Model file for the job. Use its own axes, mm. A direction names the side the tool comes from. Give positions to 0.01 mm unless a question says otherwise; leave off trailing zeros. Loops run counter-clockwise (first coordinate to the right, second up) from the corner with the lowest first, then second, coordinate; pieces in that order, holes last. Notation, with made-up numbers: M -8,45 L 15,45 A15 ccw 15,56 Z; hole C -25.75,-32.5 d11. An arc over 180 degrees is marked long. Answer in a Markdown table with one row per item.
```python
from build123d import *

# Parameters (mm, degrees)
BOSS_EXTRUDE1_DEPTH = 22.5
SKETCH2_W           = 6.85
SKETCH2_H           = 3
BOSS_EXTRUDE2_DEPTH = 10
SKETCH3_W           = 6.85
SKETCH3_H           = 3
BOSS_EXTRUDE3_DEPTH = 10
FILLET2_R           = 0.5
SKETCH5_R           = 2.01
CUT_EXTRUDE1_DEPTH  = 10


with BuildPart() as part:
    # Sketch1 → Boss-Extrude1 (new body, symmetric)
    with BuildSketch(Plane(origin=(0, 0, 0), x_dir=(1, 0, 0), z_dir=(0, 1, 0))):
        Polygon((0, 0), (-2.69457677, -2.2), (-2.69457677, 1.8), (2.55542323, 1.8), (2.55542323, -2.2), align=None)
    extrude(amount=BOSS_EXTRUDE1_DEPTH, both=True)

    # Sketch2 → Boss-Extrude2 (add)
    with BuildSketch(Plane(origin=(0, 22.5, 0), x_dir=(1, 0, 0), z_dir=(0, 1, 0))):
        with Locations((-0.06957677, 0.3)):
            Rectangle(SKETCH2_W, SKETCH2_H)
    extrude(amount=BOSS_EXTRUDE2_DEPTH)

    # Sketch3 → Boss-Extrude3 (add)
    with BuildSketch(Plane.XZ.offset(22.5)):
        with Locations((-0.06957677, -0.3)):
            Rectangle(SKETCH3_W, SKETCH3_H)
    extrude(amount=BOSS_EXTRUDE3_DEPTH)

    # Fillet2
    fillet2_edges = [part.edges().sort_by_distance(p)[0] for p in [
        (0, 0, 0),
    ]]
    fillet(fillet2_edges, radius=FILLET2_R)

    # Sketch5 → Cut-Extrude1 (cut)
    with BuildSketch(Plane(origin=(0, 0, -1.8), x_dir=(-1, 0, 0), z_dir=(0, 0, -1))):
        with Locations((0, -26.5)):
            Circle(SKETCH5_R)
        with Locations((0, 26.5)):
            Circle(SKETCH5_R)
    extrude(amount=-CUT_EXTRUDE1_DEPTH, mode=Mode.SUBTRACT)


solid = part.part
```
(1) Mould opens along Y. For faces 4 (the flat face through (2.1, 22.5, 1.6)), 5 (the cylindrical face through (0.262, -24.507, -0.321)), 6 (the flat face through (-3.495, -27, 0)), 7 (the flat face through (0, -32.5, 0)) say: pulls with the +Y half, pulls with the -Y half, needs draft (parallel to the pull), parting line crosses it, or undercut.
Established:
| item | result |
|---|---|
| face 4 | pulls with the +Y half |
| face 5 | undercut |
| face 6 | needs draft |
| face 7 | pulls with the -Y half |
(2) Saw through at C-C, the plane y = -21.5. Give the cut face in (x, z).
Established:
| item | result |
|---|---|
| outline | M -2.69,-1.8 L 2.56,-1.8 L 2.56,2.2 L 0.32,0.27 A0.5 cw -0.32,0.27 L -2.69,2.2 Z |
(3) Wall check: L1, parallel to Y at x = 0, z = 0.3; L2, parallel to Y at x = 0, z = -0.65; L3, parallel to Y at x = 1.75, z = -0.15. Give the ranges that are in metal, low to high.
Established:
| item | result |
|---|---|
| L1 | y = -32.5 to -28.51, -24.49 to -22.5, 22.5 to 24.49, 28.51 to 32.5 |
| L2 | y = -32.5 to -28.51, -24.49 to 24.49, 28.51 to 32.5 |
| L3 | y = -32.5 to -27.49, -25.51 to 25.51, 27.49 to 32.5 |
(4) Saw through at A-A, the plane y = 26.5. Give the cut face in (x, z), and give its area (3 significant figures).
Established:
| item | result |
|---|---|
| outline | M -3.49,-1.8 L -2.01,-1.8 L -2.01,1.2 L -3.49,1.2 Z; M 2.01,-1.8 L 3.36,-1.8 L 3.36,1.2 L 2.01,1.2 Z |
| area | 8.49 mm2 |
(5) Which spindle directions (+Z, -Z, +X, -X, +Y, -Y) get a long thin tool onto all of the face, cutting with end or side? Do faces 1 (the flat face through (2.1, -22.5, 1.6)), 2 (the flat face through (0, 29, 1.2)), 3 (the flat face through (0, 22.5, 1)). Say none if no direction does.
Established:
| item | result |
|---|---|
| face 1 | +Z, +X, -X, -Y |
| face 2 | +Z, +X, -X, +Y |
| face 3 | +Z |
(6) Saw through at B-B, the plane z = -0.5. Give the cut face in (x, y).
Established:
| item | result |
|---|---|
| outline | M -3.49,-32.5 L 3.36,-32.5 L 3.36,-22.5 L 2.56,-22.5 L 2.56,22.5 L 3.36,22.5 L 3.36,32.5 L -3.49,32.5 L -3.49,22.5 L -2.69,22.5 L -2.69,-22.5 L -3.49,-22.5 Z; hole C 0,-26.5 d4.02; hole C 0,26.5 d4.02 |
(7) Flat gauge pins, fed straight in: P1, Ø2.5, axis at x = 0, y = -26.5, coming from the -Z side; P2, Ø0.5, axis at x = -2.5, z = 2, coming from the -Y side. Where does each tip first touch, or does it go through?
Established:
| item | result |
|---|---|
| P1 | passes through |
| P2 | stops at y = -22.5 |
